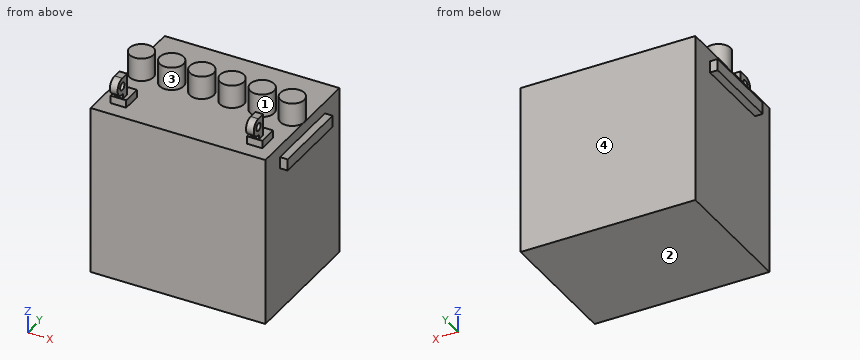
```python
from build123d import *

# Parameters (mm, degrees)
F0_W      = 226
F0_H      = 173
F1_DEPTH  = 110
F2_W      = 105
F2_H      = 15
F3_DEPTH  = 10
F4_R      = 15.5
F5_DEPTH  = 30
F6_W      = 20
F6_H      = 25
F7_DEPTH  = 10
F10_R     = 5
F11_DEPTH = 5


# Not quite as in the source:
# - a pattern or mirror of a feature is missing from the dataset's text; its kind, count and spacing are read off the source's solid


with BuildPart() as f1:
    # F0 (on Top) → F1 (new body, symmetric)
    with BuildSketch(Plane.XY):
        Rectangle(F0_W, F0_H)
    extrude(amount=F1_DEPTH, both=True)

    # F2 (on face) → F3 (join)
    with BuildSketch(Plane(origin=(-113, 0, 0), x_dir=(0, -1, 0), z_dir=(-1, 0, 0))):
        with Locations((0, 87.5)):
            Rectangle(F2_W, F2_H)
    f3 = extrude(amount=F3_DEPTH)

    # F3_copies: F3 across plane
    add(f3.mirror(Plane(origin=(0, 0, 0), x_dir=(0, 0, 1), z_dir=(1, 0, 0))))

    # F4 (on face) → F5 (join)
    with BuildSketch(Plane.XY.offset(110)):
        with BuildLine():
            ThreePointArc((-82, 4.5), (-97.5000000043, 20), (-113, 4.4999999915))
            ThreePointArc((-113, 4.4999999915), (-97.4999999957, -11), (-82, 4.5))
        make_face()
        with Locations((-58.5, 4.5)):
            Circle(F4_R)
        with Locations((-19.5, 4.5)):
            Circle(F4_R)
        with Locations((19.5, 4.5)):
            Circle(F4_R)
        with Locations((58.5, 4.5)):
            Circle(F4_R)
        with Locations((97.5, 4.5)):
            Circle(F4_R)
    extrude(amount=F5_DEPTH)

    # F6 (on face) → F7 (join)
    with BuildSketch(Plane.XY.offset(110)):
        with Locations((88, -54)):
            Rectangle(F6_W, F6_H)
    f7 = extrude(amount=F7_DEPTH)

    # F7_copies: F7 across plane
    add(f7.mirror(Plane(origin=(0, 0, 0), x_dir=(0, 0, -1), z_dir=(-1, 0, 0))))

    # F10 (on plane+point) → F11 (join, symmetric)
    with BuildSketch(Plane.YZ.offset(88)):
        with BuildLine():
            Line((-55.4758111389, 148.0241888611), (-66.5, 148.0241888611))
            ThreePointArc((-66.5, 148.0241888611), (-77.5122627569, 136.4873509794), (-65.4758111389, 126.0234897521))
            Line((-65.4758111389, 126.0234897521), (-65.4758111389, 120))
            Line((-65.4758111389, 120), (-55.4758111389, 120))
            Line((-55.4758111389, 120), (-55.4758111389, 137))
            Line((-55.4758111389, 137), (-55.4758111389, 148.0241888611))
        make_face()
        with Locations((-66.5, 137)):
            Circle(F10_R, mode=Mode.SUBTRACT)
    f11 = extrude(amount=F11_DEPTH, both=True)

    # F11_copies: F11 across plane
    add(f11.mirror(Plane(origin=(0, 0, 0), x_dir=(0, 0, -1), z_dir=(-1, 0, 0))))


solid = f1.part
```
Geometry check sheet. Reference: the model listing, model coordinates, mm. Face numbers are marked on the shaded views. A direction names the side the tool comes from. Give positions to 0.01 mm unless a question says otherwise; leave off trailing zeros. Order: outer loops, then holes, each group sorted by start corner. A loop starts at its lowest first (then second) coordinate and runs counter-clockwise, first axis right, second up. Notation, with made-up numbers: (38.5, 51.5) - (51.5, 51.5) arc R15 cw to (51.5, 67.5) - close; hole circle Ø2 at (60.5, -39). An arc over 180 degrees is marked (long way). Write item = value, one per line. Start each with the question number.
1) Access from +Z, -Z, +X, -X, +Y, -Y to the whole of each face (thin tool, end or side, straight path). Record for the marked faces 1 and 2.
2) Section check C-C (z = 41). Enter the section's corners in (x, y), then the cut area to 3 significant figures.
3) Draft check along X on the marked faces 3 and 4. Enter one of: released by +X, released by -X, zero draft, split by the parting line, or undercut.
4) Section check A-A (y = 39). Enter the section's corners in (x, z).
5) Section check D-D (x = 54.5). Enter the section's corners in (y, z).
6) Section check B-B (x = 19.5). Enter the section's corners in (y, z).
7) Scan lines: L1, parallel to Z at x = -86, y = -66; L2, parallel to X at y = -22.5, z = 68.5; L3, parallel to Z at x = 13.5, y = -3. Record each from-to range of solid material in increasing order.
8) Gauge pin test, flat ends, axial feed: pin 1 Ø1.8 at (x, z) = (-86, 124) entering from -Y; pin 2 Ø12 at (y, z) = (-29, -13.5) entering from -X; pin 3 Ø11 at (y, z) = (-61.5, 128.5) entering from +X. Record the tip position at first contact, or that the pin passes through.
Geometry check:
q1.face_1 = +Z
q1.face_2 = -Z, +X, -X, +Y, -Y
q2.outline = (-113, -86.5) - (113, -86.5) - (113, 86.5) - (-113, 86.5) - close
q2.area = 39,100 mm2
q3.face_3 = undercut
q3.face_4 = zero draft
q4.outline = (-123, 80) - (-113, 80) - (-113, -110) - (113, -110) - (113, 80) - (123, 80) - (123, 95) - (113, 95) - (113, 110) - (-113, 110) - (-113, 95) - (-123, 95) - close
q5.outline = (-86.5, -110) - (86.5, -110) - (86.5, 110) - (19.47, 110) - (19.47, 140) - (-10.47, 140) - (-10.47, 110) - (-86.5, 110) - close
q6.outline = (-86.5, -110) - (86.5, -110) - (86.5, 110) - (20, 110) - (20, 140) - (-11, 140) - (-11, 110) - (-86.5, 110) - close
q7.L1 = -110 to 120, 125.99 to 132.03, 141.97 to 148.02
q7.L2 = -113 to 113
q7.L3 = -110 to 140
q8.pin_1 = -65.48
q8.pin_2 = -113
q8.pin_3 = 93
